Could you check a few things on this model? Use its own coordinates, in mm. Round coordinates to 2 decimals unless told otherwise and drop trailing zeros. Write each loop counter-clockwise with the first axis right and the second up, starting at its lowest first coordinate (ties: lowest second). Pieces come first, ordered by that corner, then holes. Notation, with made-up numbers: M -7,31.25 L 14,31.25 A26 ccw 14,46.25 Z; hole C 85.5,42 d8. An arc over 180 degrees is marked long. One line per item, written item: value. Start each with the question number.
(1) If I drill on L1, parallel to Y at x = 0, z = 2.95; L2, parallel to Y at x = 1, z = 1.85; L3, parallel to Y at x = -6.25, z = 1.3, over which ranges is the centre line in solid material (lowest first)?
(2) I want a section at D-D on z = 2.9. Please give me the cut outline in (x, y), and give its area (3 significant figures).
(3) Thinking about a two-plate mould opening in X: for faces 1 (the face through (1.245, -2.394, 2.381)), 2 (the face through (2, -2, 3.175)), 3 (the face through (9.533, 3.002, 1.572)), which applies, released by +X, released by -X, zero draft, split by the parting line, or undercut?
(4) I'm going to push flat-ended pins straight in: pin 1 Ø1.5 at (y, z) = (3.5, 1) entering from -X; pin 2 Ø1.5 at (x, z) = (-5, 1) entering from -Y; pin 3 Ø1.5 at (x, z) = (6.5, 1.5) entering from +Y. Where does each tip first touch, or does it pass through?
(5) I want a section at A-A on y = 0. Please give me the cut outline in (x, z) (3 decimals), and give its area (3 significant figures).
(6) I want a section at C-C on z = 1.1. Please give me the cut outline in (x, y), and give its area (3 significant figures).
```python
from build123d import *

# Parameters (mm, degrees)
F0_R     = 9.9949
F0_R_2   = 2.54
F1_DEPTH = 3.175
F2_SIZE  = 2.54
F3_R     = 0.508


with BuildPart() as f1:
    # F0 (on Top) → F1 (new body)
    with BuildSketch(Plane.XY):
        Circle(F0_R)
        Circle(F0_R_2, mode=Mode.SUBTRACT)
    extrude(amount=F1_DEPTH)

    # F2
    f2_edges = [f1.edges().sort_by_distance(p)[0] for p in [
        (-2.54, 0, 0),
    ]]
    chamfer(f2_edges, length=F2_SIZE)

    # F3
    f3_edges = [f1.edges().sort_by_distance(p)[0] for p in [
        (-9.9949, 0, 3.175),
        (-9.9949, 0, 0),
    ]]
    fillet(f3_edges, radius=F3_R)


solid = f1.part
```
Found:
1. L1: y = -9.91 to -2.54, 2.54 to 9.91
1. L2: y = -9.94 to -3.07, 3.07 to 9.94
1. L3: y = -7.8 to 7.8
2. outline: C 0,0 d19.88; hole C 0,0 d5.08
2. area: 290 mm²
3. face 1: undercut
3. face 2: zero draft
3. face 3: split by the parting line
4. pin 1: stops at x = -9.61
4. pin 2: stops at y = -9.05
4. pin 3: stops at y = 8.18
5. outline: M -9.995,0.508 A0.508 ccw -9.487,0 L -5.08,0 L -2.54,2.54 L -2.54,3.175 L -9.487,3.175 A0.508 ccw -9.995,2.667 Z; M 2.54,2.54 L 5.08,0 L 9.487,0 A0.508 ccw 9.995,0.508 L 9.995,2.667 A0.508 ccw 9.487,3.175 L 2.54,3.175 Z
5. area: 40.7 mm²
6. outline: C 0,0 d19.99; hole C 0,0 d7.96
6. area: 264 mm²
